```python
from build123d import *

# Parameters (mm, degrees)
SKETCH1_W                      = 129.93
SKETCH1_H                      = 79.93
BOSS_EXTRUDE1_DEPTH            = 1.2
FILLET1_R                      = 3.175
CUT_EXTRUDE2_REACH             = 78.283
SKETCH3_R                      = 2
CUT_EXTRUDE1_REACH             = 78.283
SKETCH2_R                      = 1.25
CUT_EXTRUDE1_DIRECTION_2_DEPTH = 77.282976148
BOSS_EXTRUDE2_START            = 5
SKETCH4_R                      = 3.5
SKETCH4_R_2                    = 1.25
BOSS_EXTRUDE2_DEPTH            = 5


with BuildPart() as part:
    # Sketch1 → Boss-Extrude1 (new body)
    with BuildSketch(Plane.XY):
        Rectangle(SKETCH1_W, SKETCH1_H)
    extrude(amount=BOSS_EXTRUDE1_DEPTH)

    # Fillet1
    fillet1_edges = [part.edges().sort_by_distance(p)[0] for p in [
        (64.965, -39.965, 0.6),
        (-64.965, -39.965, 0.6),
        (-64.965, 39.965, 0.6),
        (64.965, 39.965, 0.6),
    ]]
    fillet(fillet1_edges, radius=FILLET1_R)

    # Sketch3 → Cut-Extrude2 (cut, up to next)
    with BuildSketch(Plane.XY.offset(1.2), mode=Mode.PRIVATE) as cut_extrude2_sk1:
        with Locations((-50, 0)):
            Circle(SKETCH3_R)
    cut_extrude2_tool1 = extrude(cut_extrude2_sk1.sketch, amount=-CUT_EXTRUDE2_REACH, mode=Mode.PRIVATE) & part.part
    # Sketch3 → Cut-Extrude2 (cut, up to next)
    with BuildSketch(Plane.XY.offset(1.2), mode=Mode.PRIVATE) as cut_extrude2_sk2:
        with Locations(Location((50, 0, 0), (0, 0, 180))):
            Circle(SKETCH3_R)
    cut_extrude2_tool2 = extrude(cut_extrude2_sk2.sketch, amount=-CUT_EXTRUDE2_REACH, mode=Mode.PRIVATE) & part.part
    add(cut_extrude2_tool1.solids().sort_by_distance((-50, 0, 1.2))[0], mode=Mode.SUBTRACT)
    add(cut_extrude2_tool2.solids().sort_by_distance((50, 0, 1.2))[0], mode=Mode.SUBTRACT)

    # Sketch2 → Cut-Extrude1 (cut, up to next)
    with BuildSketch(Plane.XY.offset(1.2), mode=Mode.PRIVATE) as cut_extrude1_sk1:
        with Locations(Location((-8.156928596, -26.04, 0), (0, 0, 180))):
            Circle(SKETCH2_R)
    cut_extrude1_tool1 = extrude(cut_extrude1_sk1.sketch, amount=-CUT_EXTRUDE1_REACH, mode=Mode.PRIVATE) & part.part
    # Sketch2 → Cut-Extrude1 (cut, up to next)
    with BuildSketch(Plane.XY.offset(1.2), mode=Mode.PRIVATE) as cut_extrude1_sk2:
        with Locations(Location((37.693071404, 0, 0), (0, 0, 180))):
            Circle(SKETCH2_R)
    cut_extrude1_tool2 = extrude(cut_extrude1_sk2.sketch, amount=-CUT_EXTRUDE1_REACH, mode=Mode.PRIVATE) & part.part
    add(cut_extrude1_tool1.solids().sort_by_distance((-8.156929, -26.04, 1.2))[0], mode=Mode.SUBTRACT)
    add(cut_extrude1_tool2.solids().sort_by_distance((37.693071, 0, 1.2))[0], mode=Mode.SUBTRACT)

    # Sketch2 → Cut-Extrude1 direction 2 (cut)
    with BuildSketch(Plane.XY.offset(1.2)):
        with Locations(Location((-8.156928596, -26.04, 0), (0, 0, 180))):
            Circle(SKETCH2_R)
        with Locations(Location((37.693071404, 0, 0), (0, 0, 180))):
            Circle(SKETCH2_R)
    extrude(amount=CUT_EXTRUDE1_DIRECTION_2_DEPTH, mode=Mode.SUBTRACT)

    # Sketch4 → Boss-Extrude2 (add)
    # profile 1 of 2: a face of its own
    with BuildSketch(Plane.XY.offset(1.2).offset(BOSS_EXTRUDE2_START)):
        with Locations(Location((-8.156928596, -26.04, 0), (0, 0, 180))):
            Circle(SKETCH4_R)
        with Locations(Location((-8.156928596, -26.04, 0), (0, 0, 180))):
            Circle(SKETCH4_R_2, mode=Mode.SUBTRACT)
    # profile 2 of 2: a face of its own
    with BuildSketch(Plane.XY.offset(1.2).offset(BOSS_EXTRUDE2_START)):
        with Locations(Location((37.693071404, 0, 0), (0, 0, 180))):
            Circle(SKETCH4_R)
        with Locations(Location((37.693071404, 0, 0), (0, 0, 180))):
            Circle(SKETCH4_R_2, mode=Mode.SUBTRACT)
    extrude(amount=-BOSS_EXTRUDE2_DEPTH)


solid = part.part
```
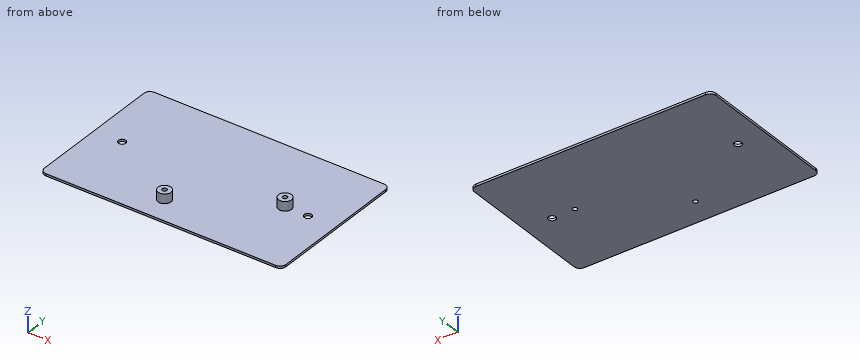
Here's how the part is built. I have some questions about the finished solid (model axes, mm). Give positions to 0.01 mm unless a question says otherwise; leave off trailing zeros. Order: outer loops, then holes, each group sorted by start corner. A loop starts at its lowest first (then second) coordinate and runs counter-clockwise, first axis right, second up. Notation, with made-up numbers: M 43.25,45.25 L 77.25,45.25 A6 ccw 77.25,56.25 Z; hole C 87,-37 d11. An arc over 180 degrees is marked long. Use a Markdown table: item, result. Add a question column.
1. Suppose I cut it at D-D (y = 0). List the corners of the cut face in (x, z) for me (3 decimals), and give its area (3 significant figures).
2. Suppose I cut it at C-C (z = 5). List the corners of the cut face in (x, y) for me.
3. Suppose I cut it at B-B (y = -26.04). List the corners of the cut face in (x, z) for me (3 decimals).
4. For pin 1 Ø2 at (x, y) = (-8.16, -26.04) entering from +Z, with a flat end and sliding along its axis, tell me the tip position at first contact or that it passes through.
5. Suppose I cut it at A-A (x = 50). List the corners of the cut face in (y, z) for me (3 decimals).
6. I need wall thicknesses on probe 1 along Y at (x, z) = (-50, 0.35) (3 decimals); probe 2 along X at (y, z) = (-26.04, 4.5); probe 3 along Z at (x, y) = (50, 15). Which ranges of each line are inside material? Lowest first, please. Write a range as from..to.
Results list:
| question | item | result |
|---|---|---|
| 1 | outline | M -64.965,0 L -52,0 L -52,1.2 L -64.965,1.2 Z; M -48,0 L 36.443,0 L 36.443,6.2 L 34.193,6.2 L 34.193,1.2 L -48,1.2 Z; M 38.943,0 L 48,0 L 48,1.2 L 41.193,1.2 L 41.193,6.2 L 38.943,6.2 Z; M 52,0 L 64.965,0 L 64.965,1.2 L 52,1.2 Z |
| 1 | area | 166 mm² |
| 2 | outline | C -8.16,-26.04 d7; C 37.69,0 d7; hole C -8.16,-26.04 d2.5; hole C 37.69,0 d2.5 |
| 3 | outline | M -64.965,0 L -9.407,0 L -9.407,6.2 L -11.657,6.2 L -11.657,1.2 L -64.965,1.2 Z; M -6.907,0 L 64.965,0 L 64.965,1.2 L -4.657,1.2 L -4.657,6.2 L -6.907,6.2 Z |
| 4 | pin 1 | passes through |
| 5 | outline | M -39.965,0 L -2,0 L -2,1.2 L -39.965,1.2 Z; M 2,0 L 39.965,0 L 39.965,1.2 L 2,1.2 Z |
| 6 | probe 1 | y = -39.965..-2, 2..39.965 |
| 6 | probe 2 | x = -11.66..-9.41, -6.91..-4.66 |
| 6 | probe 3 | z = 0..1.2 |
